from build123d import *

# Parameters (mm, degrees)
BOSS_EXTRUDE1_DEPTH = 41.5
CUT_EXTRUDE1_START  = 41.5
SKETCH1_3_R         = 2.1
CUT_EXTRUDE1_DEPTH  = 84.704514495


with BuildPart() as part:
    # Sketch1 → Boss-Extrude1 (new, symmetric)
    with BuildSketch(Plane(origin=(0, 0, 0), x_dir=(1, 0, 0), z_dir=(0, 1, 0))):
        Polygon((5.065112622, 2.770914552), (0.132873917, 5.77197348), (-4.932238705, 3.001058928), (-5.065112622, -2.770914552), (-0.132873917, -5.77197348), (4.932238705, -3.001058928), align=None)
    extrude(amount=BOSS_EXTRUDE1_DEPTH, both=True)

    # Sketch1_3 → Cut-Extrude1 (cut, through all)
    with BuildSketch(Plane(origin=(0, 0, 0), x_dir=(1, 0, 0), z_dir=(0, 1, 0)).offset(CUT_EXTRUDE1_START)):
        with Locations(Location((0, 0, 0), (0, 0, 270))):
            Circle(SKETCH1_3_R)
    extrude(amount=-CUT_EXTRUDE1_DEPTH, mode=Mode.SUBTRACT)


solid = part.part
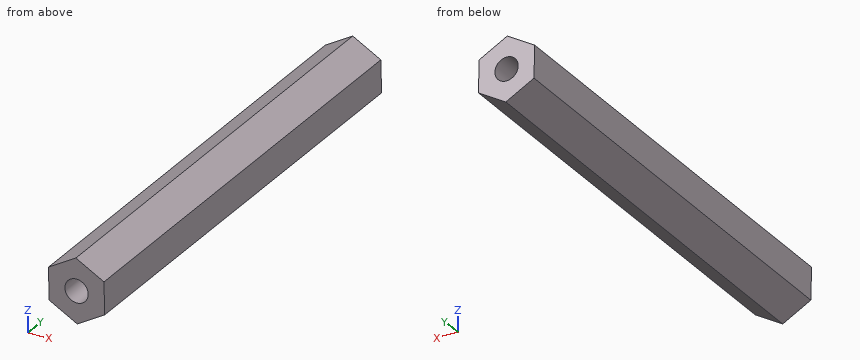
Design review of the part built by this model. Coordinates are the model's own, in mm. Coordinates: 2 decimals unless noted, no trailing zeros. Order: outer loops, then holes, each group sorted by start corner. A loop starts at its lowest first (then second) coordinate and runs counter-clockwise, first axis right, second up. Notation, with made-up numbers: (40, -16.75) -> (78, -16.75) arc R16 cw to (78, 10.25) -> close; hole circle Ø11 at (73, -29.75). An arc over 180 degrees is marked (long way). One line per item, written item: value.
1) We need section C-C, the plane x = -3.25. Give the boundary of the cut face in (y, z), then the cut area to 3 significant figures.
Output values:
outline: (-41.5, -3.92) -> (41.5, -3.92) -> (41.5, 3.88) -> (-41.5, 3.88) -> close
area: 647 mm2
2) We need section A-A, the plane y = -35.5. Give the boundary of the cut face in (x, z).
Output values:
outline: (-5.07, 2.77) -> (-4.93, -3) -> (0.13, -5.77) -> (5.07, -2.77) -> (4.93, 3) -> (-0.13, 5.77) -> close; hole circle Ø4.2 at (0, 0)
3) To check wall thickness, follow probe 1 along Z at (x, y) = (1.75, -28.5); probe 2 along Z at (x, y) = (0.5, 21); probe 3 along X at (y, z) = (-12, 0). State the ranges of each line that lie inside material, in increasing order. Write a range as [from, to].
Output values:
probe 1: z = [-4.79, -1.16], [1.16, 4.74]
probe 2: z = [-5.55, -2.04], [2.04, 5.43]
probe 3: x = [-5, -2.1], [2.1, 5]
4) We need section D-D, the plane z = 4. Give the boundary of the cut face in (x, y), then the cut area to 3 significant figures.
Output values:
outline: (-3.05, -41.5) -> (3.11, -41.5) -> (3.11, 41.5) -> (-3.05, 41.5) -> close
area: 511 mm2
5) Clearance check with flat-ended pins moving along their axes: P1, Ø2, axis at x = -3.5, y = -26, coming from the +Z side; P2, Ø4, axis at x = 1.5, y = 5, coming from the -Z side; P3, Ø6, axis at x = 0.5, y = 28.5, coming from the +Z side; P4, Ø4, axis at x = 4, y = -22, coming from the -Z side. State where each tip first meets the part, or that it passes through.
Output values:
P1: stops at z = 4.33
P2: stops at z = -5.77
P3: stops at z = 5.77
P4: stops at z = -4.64
6) We need section B-B, the plane z = 0. Give the boundary of the cut face in (x, y), then the cut area to 3 significant figures.
Output values:
outline: (-5, -41.5) -> (-2.1, -41.5) -> (-2.1, 41.5) -> (-5, 41.5) -> close; (2.1, -41.5) -> (5, -41.5) -> (5, 41.5) -> (2.1, 41.5) -> close
area: 482 mm2
